Print and shaded views of the part. All mm, measured from the part's lowest x, y and z. Coordinates: 2 decimals unless noted, no trailing zeros. Loops run counter-clockwise (first coordinate to the right, second up) from the corner with the lowest first, then second, coordinate; pieces in that order, holes last. Notation, with made-up numbers: M 14.25,10.25 L 72.25,10.25 A24 cw 72.25,20.25 Z; hole C -22.5,-16 d7. An arc over 180 degrees is marked long. Answer as a JSON object with one key per item and string values. Group by question number.
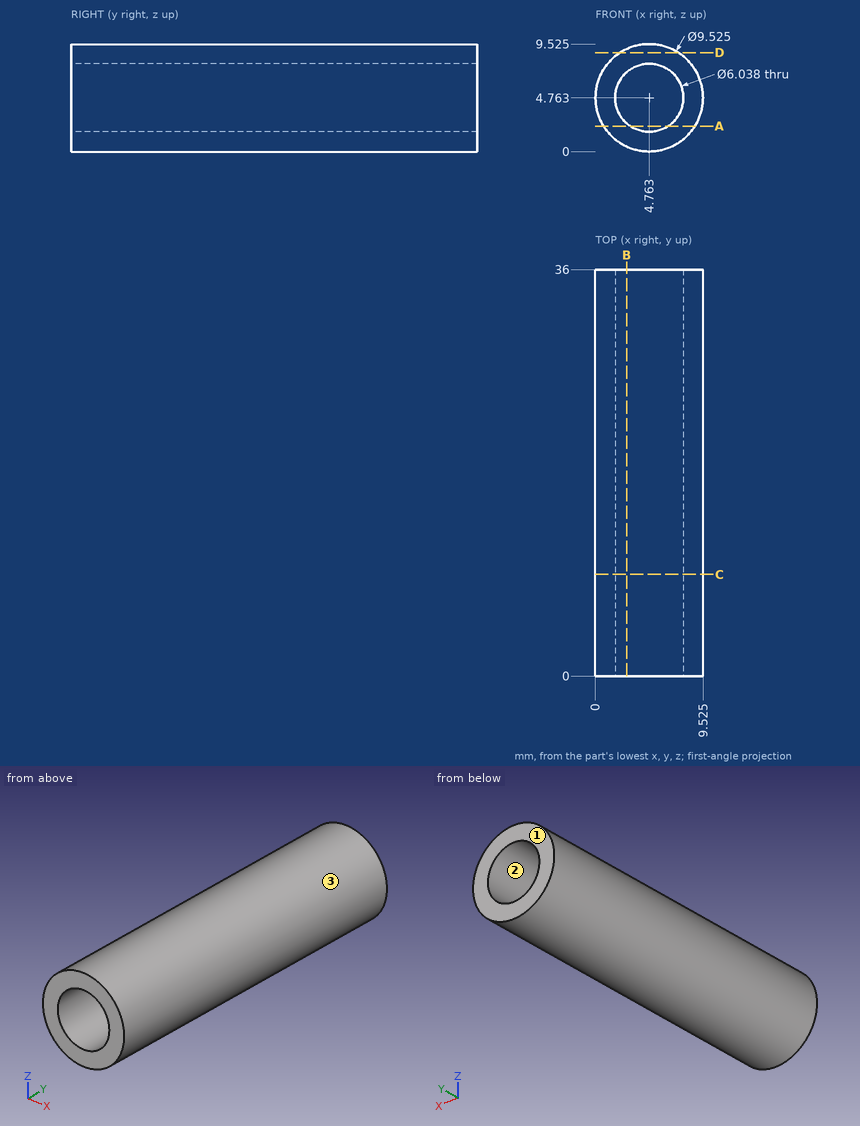
Item 1: Slice it at A-A, the plane z = 2.25. Write the cut outline in (x, y).
Item 2: Drill centre lines: L1, parallel to Z at x = 4.75, y = 24 (1 decimal); L2, parallel to Z at x = 7, y = 15 (1 decimal); L3, parallel to X at y = 26.5, z = 3.5 (1 decimal). Where is each one in solid material? Low to high. Write a range as from..to.
Item 3: Slice it at D-D, the plane z = 8.75. Write the cut outline in (x, y).
Item 4: Slice it at B-B, the plane x = 2.75. Write the cut outline in (y, z), then the cut area to 3 significant figures.
Item 5: Pull direction Z, two halves, no side cores. Call the marked faces 1, 2 and 3: released by +Z, released by -Z, zero draft, split by the parting line, or undercut.
Item 6: Pin check, flat tips, straight feed: pin 1 (3 mm diameter, centred on y = 29, z = 2, fed in from +X) (1 decimal); pin 2 (4 mm diameter, centred on y = 23, z = 7.5, fed in from +X). Stop position of each tip, or through.
Item 7: Slice it at C-C, the plane y = 9. Write the cut outline in (x, z) (1 decimal).
Computed:
{
 "1": {"outline": "M 0.72,0 L 3.09,0 L 3.09,36 L 0.72,36 Z; M 6.44,0 L 8.81,0 L 8.81,36 L 6.44,36 Z"},
 "2": {"L1": "0..1.7, 7.8..9.5", "L2": "0.6..2.7, 6.8..9", "L3": "0.2..2, 7.5..9.4"},
 "3": {"outline": "M 2.16,0 L 7.37,0 L 7.37,36 L 2.16,36 Z"},
 "4": {"outline": "M 0,0.45 L 36,0.45 L 36,2.51 L 0,2.51 Z; M 0,7.01 L 36,7.01 L 36,9.08 L 0,9.08 Z", "area": "149 mm2"},
 "5": {"face 1": "zero draft", "face 2": "undercut", "face 3": "split by the parting line"},
 "6": {"pin 1": "x = 9.4", "pin 2": "x = 9.47"},
 "7": {"outline": "C 4.8,4.8 d9.5; hole C 4.8,4.8 d6"}
}
